```python
from build123d import *

# Parameters (mm, degrees)
SKETCH_1_W          = 145
SKETCH_1_H          = 61.5
SKETCH_1_R          = 2
EXTRUDE_1_DEPTH     = 3
FILLET_1_R          = 3
SKETCH_4_W          = 105
SKETCH_4_H          = 20
CUT_EXTRUDE_3_DEPTH = 6
SKETCH_6_R          = 1.5
CUT_EXTRUDE_6_DEPTH = 83.378698703
FILLET_3_R          = 3


with BuildPart() as part:
    # 草图1 → 凸台-拉伸1 (new body)
    with BuildSketch(Plane(origin=(0, 0, 0), x_dir=(1, 0, 0), z_dir=(0, 1, 0))):
        with Locations((0, -8.25)):
            Rectangle(SKETCH_1_W, SKETCH_1_H)
        with Locations(Location((-67.5, 12.5, 0), (0, 0, 270))):
            Circle(SKETCH_1_R, mode=Mode.SUBTRACT)
        with Locations(Location((-67.5, -12.5, 0), (0, 0, 270))):
            Circle(SKETCH_1_R, mode=Mode.SUBTRACT)
        with Locations(Location((67.5, 12.5, 0), (0, 0, 270))):
            Circle(SKETCH_1_R, mode=Mode.SUBTRACT)
        with Locations(Location((67.5, -12.5, 0), (0, 0, 270))):
            Circle(SKETCH_1_R, mode=Mode.SUBTRACT)
        with Locations(Location((15, 12.5, 0), (0, 0, 270))):
            Circle(SKETCH_1_R, mode=Mode.SUBTRACT)
        with Locations(Location((15, -12.5, 0), (0, 0, 270))):
            Circle(SKETCH_1_R, mode=Mode.SUBTRACT)
        with Locations(Location((-47.5, 12.5, 0), (0, 0, 270))):
            Circle(SKETCH_1_R, mode=Mode.SUBTRACT)
        with Locations(Location((-47.5, -12.5, 0), (0, 0, 270))):
            Circle(SKETCH_1_R, mode=Mode.SUBTRACT)
        with Locations(Location((47.5, 12.5, 0), (0, 0, 270))):
            Circle(SKETCH_1_R, mode=Mode.SUBTRACT)
        with Locations(Location((47.5, -12.5, 0), (0, 0, 270))):
            Circle(SKETCH_1_R, mode=Mode.SUBTRACT)
    extrude(amount=EXTRUDE_1_DEPTH)

    # 圆角1
    fillet_1_edges = [part.edges().sort_by_distance(p)[0] for p in [
        (72.5, 1.5, -22.5),
        (72.5, 1.5, 39),
        (-72.5, 1.5, 39),
        (-72.5, 1.5, -22.5),
    ]]
    fillet(fillet_1_edges, radius=FILLET_1_R)

    # 草图4 → 切除-拉伸3 (cut)
    with BuildSketch(Plane(origin=(0, 3, 0), x_dir=(1, 0, 0), z_dir=(0, 1, 0))):
        with Locations((0, -29)):
            Rectangle(SKETCH_4_W, SKETCH_4_H)
    extrude(amount=-CUT_EXTRUDE_3_DEPTH, mode=Mode.SUBTRACT)

    # 草图6 → 切除-拉伸6 (cut, through all)
    with BuildSketch(Plane(origin=(0, 3, 0), x_dir=(1, 0, 0), z_dir=(0, 1, 0))):
        with Locations(Location((-30.2, 0.5, 0), (0, 0, 270))):
            Circle(SKETCH_6_R)
        with Locations(Location((-10.2, 0.5, 0), (0, 0, 270))):
            Circle(SKETCH_6_R)
        with Locations(Location((9.8, 0.5, 0), (0, 0, 270))):
            Circle(SKETCH_6_R)
        with Locations(Location((29.8, 0.5, 0), (0, 0, 270))):
            Circle(SKETCH_6_R)
    extrude(amount=-CUT_EXTRUDE_6_DEPTH, mode=Mode.SUBTRACT)

    # 圆角3
    fillet_3_edges = [part.edges().sort_by_distance(p)[0] for p in [
        (52.5, 1.5, 39),
        (-52.5, 1.5, 39),
        (-52.5, 1.5, 19),
        (52.5, 1.5, 19),
    ]]
    fillet(fillet_3_edges, radius=FILLET_3_R)


solid = part.part
```
Read the model definition and answer for the solid it produces. Units are mm, in the model's axes. A direction names the side the tool comes from. Coordinates: 2 decimals unless noted, no trailing zeros. Loops run counter-clockwise (first coordinate to the right, second up) from the corner with the lowest first, then second, coordinate; pieces in that order, holes last.
(1) The part is cut by section A-A (x = -67.5). Determine the outline of the cut face in (y, z).
Solution:
outline: (0, -22.5) - (3, -22.5) - (3, -14.5) - (0, -14.5) - close; (0, -10.5) - (3, -10.5) - (3, 10.5) - (0, 10.5) - close; (0, 14.5) - (3, 14.5) - (3, 39) - (0, 39) - close
(2) A tool of negligible diameter and unlimited length cuts with its end or side. For faces 5 (the face through (52.5, 2, 29)), 6 (the face through (62, 1, 39)), from which of +Z, -Z, +X, -X, +Y, -Y can it reach the whole face along a straight path? Write none if from no direction.
Solution:
face 5: +Z, +Y, -Y
face 6: +Z, +X, -X, +Y, -Y
(3) The part is cut by section D-D (z = -0.5). Determine the outline of the cut face in (x, y), and give its area (3 significant figures).
Solution:
outline: (-72.5, 0) - (-31.7, 0) - (-31.7, 3) - (-72.5, 3) - close; (-28.7, 0) - (-11.7, 0) - (-11.7, 3) - (-28.7, 3) - close; (-8.7, 0) - (8.3, 0) - (8.3, 3) - (-8.7, 3) - close; (11.3, 0) - (28.3, 0) - (28.3, 3) - (11.3, 3) - close; (31.3, 0) - (72.5, 0) - (72.5, 3) - (31.3, 3) - close
area: 399 mm2
(4) Consider line 1 along X through (y, z) = (0.9, -12.5); line 2 along X through (y, z) = (2.35, -0.5); line 3 along X through (y, z) = (2.55, 32). Determine where each line is inside the solid, lowest interval first.
Solution:
line 1: x = -72.5 to -69.5, -65.5 to -49.5, -45.5 to 13, 17 to 45.5, 49.5 to 65.5, 69.5 to 72.5
line 2: x = -72.5 to -31.7, -28.7 to -11.7, -8.7 to 8.3, 11.3 to 28.3, 31.3 to 72.5
line 3: x = -72.5 to -52.5, 52.5 to 72.5
(5) The part is cut by section C-C (y = 2.2). Count the separate pieces of the cut face and the enclosed holes in it, and give its area (3 significant figures).
Solution:
separate pieces: 1
enclosed holes: 14
area: 6,660 mm2
(6) The part is cut by section B-B (z = 12.5). Determine the outline of the cut face in (x, y).
Solution:
outline: (-72.5, 0) - (-69.5, 0) - (-69.5, 3) - (-72.5, 3) - close; (-65.5, 0) - (-49.5, 0) - (-49.5, 3) - (-65.5, 3) - close; (-45.5, 0) - (13, 0) - (13, 3) - (-45.5, 3) - close; (17, 0) - (45.5, 0) - (45.5, 3) - (17, 3) - close; (49.5, 0) - (65.5, 0) - (65.5, 3) - (49.5, 3) - close; (69.5, 0) - (72.5, 0) - (72.5, 3) - (69.5, 3) - close
(7) The mould has two halves that part along X. Classify faces 1 (the face through (31.287, 1.521, -0.695)), 2 (the face through (8.336, 1.521, -0.825)), 3 (the face through (-1, 0, 1)), 4 (the face through (-71.64, 1.52, 38.1)): released by +X, released by -X, zero draft, split by the parting line, or undercut.
Solution:
face 1: undercut
face 2: undercut
face 3: zero draft
face 4: released by -X
